Autodesk Inventor part; units mm, degrees
ref_plane "YZ Plane" through (0, 0, 0) normal (1, 0, 0) x (0, 1, 0)
ref_plane "XZ Plane" through (0, 0, 0) normal (0, 1, 0) x (-1, 0, 0)
ref_plane "XY Plane" through (0, 0, 0) normal (0, 0, 1) x (1, 0, 0)
sketch "Эскиз1" plane through (0, 0, 0) normal (0, 1, 0) x (-1, 0, 0)
  line L0 (0, 94.5239) -> (-30, 94.5239)
  line L1 (-30, 94.5239) -> (-30, -95.4761)
  line L2 (-30, -95.4761) -> (0, -95.4761)
  line L3 (0, -95.4761) -> (0, 94.5239)
  line L4 (-30, 50.5239) -> (2, 50.5239)
  line L5 (2, 50.5239) -> (2, -51.4761)
  line L6 (2, -51.4761) -> (-30, -51.4761)
  line L7 (-30, -51.4761) -> (-30, 50.5239)
  point P0 (0, 0)
  point P1 (0, -51.4761)
  point P2 (0, 50.5239)
  dimension "d0" = 190
  dimension "d2" = 30
  dimension "d3" = 32
  dimension "d4" = 44
  dimension "d13" = 44
extrude "Выдавливание1" add sketch "Эскиз1" along normal blind 400
sketch "Эскиз2" plane through (-2, 0, -51.4761) normal (-1, 0, 0) x (0, 0, 1)
  line L0 (25, -29) -> (77, -29)
  line L1 (77, -29) -> (77, 456)
  line L2 (77, 456) -> (25, 456)
  line L3 (25, 456) -> (25, -29)
  line L4 (0, 0) -> (102, 0)
  line L5 (102, 0) -> (102, 400)
  line L6 (0, 400) -> (102, 400)
  line L7 (0, 0) -> (0, 400)
  point P0 (51.4761, 0)
  point P1 (77, 400)
  point P2 (25, 400)
  point P3 (25, 0)
  point P4 (77, 0)
  dimension "d8" = 25
  dimension "d9" = 25
  dimension "d10" = 52
extrude "Выдавливание2" cut sketch "Эскиз2" against normal blind 7.4 contours L3 L6 L1 L4
sketch "Эскиз3" plane through (-2, 0, 50.5239) normal (-1, 0, 0) x (0, 0, 1)
  line L0 (44, 0) -> (44, 400)
  line L1 (-146, 0) -> (-146, 400)
  line L2 (44, 130.4195) -> (-146, 130.4195)
  line L3 (-146, 130.4195) -> (-146, 122.295)
  line L4 (-146, 122.295) -> (44, 122.295)
  line L5 (44, 122.295) -> (44, 130.4195)
  line L6 (-25, 400) -> (-25, 0)
  line L7 (-25, 0) -> (0, 0)
  line L8 (0, 0) -> (0, 400)
  line L9 (-25, 400) -> (0, 400)
  line L10 (-77, 0) -> (-77, 400)
  line L11 (-102, 400) -> (-77, 400)
  line L12 (-102, 0) -> (-102, 400)
  line L13 (-102, 0) -> (-77, 0)
  point P0 (-50.5239, 0)
  point P1 (0, 130.4195)
  point P2 (0, 122.295)
  point P3 (-102, 122.295)
  point P4 (-102, 130.4195)
extrude "Выдавливание3" add sketch "Эскиз3" against normal blind 10 contours L4 L8 L2 L0 | L4 L1 L2 L12
sketch "Эскиз4" plane through (5.4, 0, -51.4761) normal (-1, 0, 0) x (0, 0, 1)
  line L0 (76.5, 183) -> (25.5, 183)
  line L1 (76.5, 222) -> (76.5, 183)
  line L2 (25.5, 222) -> (76.5, 222)
  line L3 (25.5, 183) -> (25.5, 222)
  circle A0 centre (71, 190.5) radius 2.75
  circle A1 centre (31, 190.5) radius 2.75
  circle A2 centre (31, 214.5) radius 2.75
  circle A3 centre (71, 214.5) radius 2.75
  line L4 (76, 263) -> (77, 263)
  line L5 (76.5, 263) -> (76.5, 222)
  line L6 (76.5, 263) -> (25.5, 263)
  line L7 (76.5, 302) -> (76.5, 263)
  line L8 (25.5, 302) -> (76.5, 302)
  line L9 (25.5, 263) -> (25.5, 302)
  circle A4 centre (71, 270.5) radius 2.75
  circle A5 centre (31, 270.5) radius 2.75
  circle A6 centre (31, 294.5) radius 2.75
  circle A7 centre (71, 294.5) radius 2.75
  point P0 (51.4761, 0)
  point P1 (51, 182.5)
  point P2 (51, 262.5)
extrude "Выдавливание4" cut sketch "Эскиз4" against normal blind 33 contours A0 | A1 | A2 | A3 | A4 | A5 | A6 | A7
properties part number "Zplita"
Design review of the part built by this model. Coordinates are the model's own, in mm. A direction names the side the tool comes from. Round coordinates to 2 decimals unless told otherwise and drop trailing zeros. Write each loop counter-clockwise with the first axis right and the second up, starting at its lowest first coordinate (ties: lowest second). Pieces come first, ordered by that corner, then holes. Notation, with made-up numbers: (55, 56.5) -> (59, 56.5) arc R29 cw to (59, 88.5) -> close; hole circle Ø1 at (-33.5, 39.5). An arc over 180 degrees is marked (long way). One line per item, written item: value. Start each with the question number.
Q1. Insertion check: P1, Ø1, axis at x = -1.5, y = 88.5, coming from the +Z side; P2, Ø0.6, axis at x = -1, z = -74, coming from the -Y side (3 decimals); P3, Ø9, axis at y = 190.5, z = 19.52, coming from the -X side; P4, Ø4.5, axis at y = 214.5, z = 19.52, coming from the -X side. Each pin has a flat end and moves straight along its axis. Give the tip position at first contact, or say it passes through.
Q2. Add section B-B (z = 55.5). Give the boundary of the cut face in (x, y) (1 decimal), then the cut area to 3 significant figures.
Q3. Add section C-C (z = -10.5). Give the boundary of the cut face in (x, y), then the cut area to 3 significant figures.
Q4. The part is to be moulded in two halves that separate along Z. For faces 4 (the face through (17, 197, 94.524)), 5 (the face through (2, 203, -26.476)), 6 (the face through (0, 263, -74)), 7 (the face through (5.4, 203, -1)), say which applies: pulls with the +Z half, pulls with the -Z half, needs draft (parallel to the pull), parting line crosses it, or undercut.
Q5. Add section A-A (y = 347.5). Give the boundary of the cut face in (x, z).
Q6. To check wall thickness, follow probe 1 along Z at (x, y) = (17.75, 294.5); probe 2 along Z at (x, y) = (18, 294); probe 3 along Z at (x, y) = (2, 24). State the ranges of each line that lie inside material, in increasing order.
Q7. Tool access review of faces 1 (the face through (0, 60, 72)), 2 (the face through (2, 197, 25.524)), 3 (the face through (0, 60, -74)): name each direction out of +Z, -Z, +X, -X, +Y, -Y from which nothing blocks a thin tool from reaching the whole face with its end or side.
Response:
1. P1: stops at z = 50.52
1. P2: stops at y = 122.295
1. P3: stops at x = 5.4
1. P4: passes through
2. outline: (-2, 122.3) -> (0, 122.3) -> (0, 0) -> (30, 0) -> (30, 400) -> (0, 400) -> (0, 130.4) -> (-2, 130.4) -> close
2. area: 12,000 mm^2
3. outline: (5.4, 0) -> (30, 0) -> (30, 400) -> (5.4, 400) -> close
3. area: 9,840 mm^2
4. face 4: pulls with the +Z half
4. face 5: undercut
4. face 6: needs draft
4. face 7: undercut
5. outline: (-2, -51.48) -> (0, -51.48) -> (0, -95.48) -> (30, -95.48) -> (30, 94.52) -> (0, 94.52) -> (0, 50.52) -> (-2, 50.52) -> (-2, 25.52) -> (5.4, 25.52) -> (5.4, -26.48) -> (-2, -26.48) -> close
6. probe 1: z = -95.48 to -23.23, -17.73 to 16.77, 22.27 to 94.52
6. probe 2: z = -95.48 to -23.18, -17.77 to 16.82, 22.23 to 94.52
6. probe 3: z = -95.48 to -26.48, 25.52 to 94.52
7. face 1: +Z, -X, -Y
7. face 2: -X, +Y, -Y
7. face 3: -Z, -X, -Y
